Input: dimensioned drawing with shaded views. Units: mm. Origin: part minimum x, y, z. A direction names the side the tool comes from. Coordinates: 2 decimals unless noted, no trailing zeros.
(1) Line query: L1, parallel to Y at x = 33.5, z = 50; L2, parallel to Z at x = 90, y = 7.75 (1 decimal). Output: solid intervals per line, ascending.
(2) Contact query for a flat-ended pin moving along its axis: P1, Ø7, axis at x = 107.5, z = 51.5, coming from the +Y side. Output: stop coordinate, or through.
(3) Set-up query: the marked faces 1 and 2. Return all of +Z, -Z, +X, -X, +Y, -Y with unobstructed straight access to the full face (end or side cutting, diameter ignored); none if empty.
(4) Mould query, pull axis Z, two halves, no side actions, for the marked faces 3, 4, 5 and 6. Classes: released by +Z, released by -Z, zero draft, split by the parting line, or undercut.
(5) Section B-B, the plane y = 11. Give the number of separate pieces and of enclosed holes in the cut face, then the cut area to 3 significant figures.
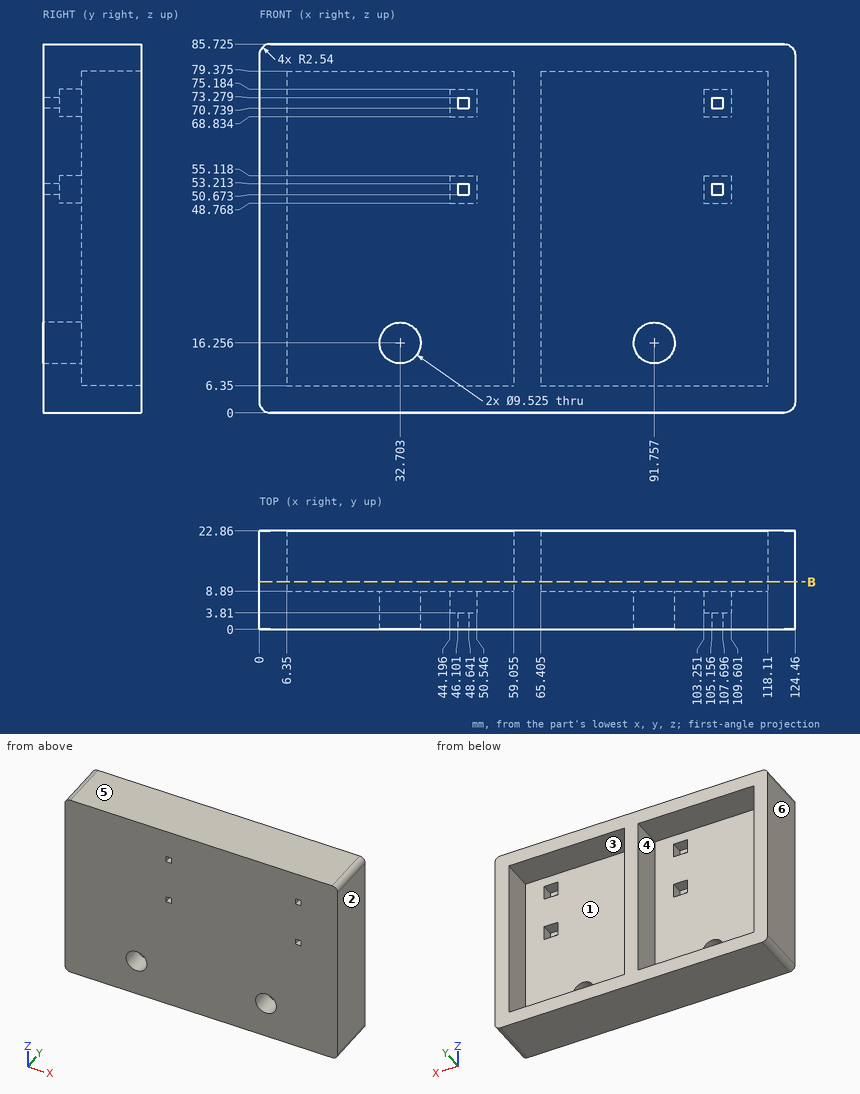
Report:
1. L1: y = 0 to 8.89
1. L2: z = 0 to 11.8, 20.7 to 85.7
2. P1: stops at y = 8.89
3. face 1: +Y
3. face 2: +Z, -Z, +X, +Y, -Y
4. face 3: undercut
4. face 4: undercut
4. face 5: released by +Z
4. face 6: zero draft
5. separate pieces: 1
5. enclosed holes: 2
5. area: 2,970 mm2
